```python
from build123d import *

# Parameters (mm, degrees)
BOSS_EXTRUDE1_DEPTH   = 7.9375
FILLET1_R             = 7.9375
SKETCH6_W             = 3.175
SKETCH6_H             = 7.9375
BOSS_EXTRUDE2_DEPTH   = 12.7
FILLET2_R             = 4.1275
FILLET3_R             = 4.1275
F_6_CLEARANCE_HOLE1_D = 4.3053


# Some blends are built 0.0001 mm under size
with BuildPart() as part:
    # Sketch1 → Boss-Extrude1 (new body)
    with BuildSketch(Plane(origin=(0, 0, 0), x_dir=(1, 0, 0), z_dir=(0, 1, 0))):
        Polygon((0, 0), (0, 22.225), (7.9375, 22.225), (7.9375, 50.45837), (11.1125, 50.45837), (11.1125, 19.05), (3.175, 19.05), (3.175, 0), align=None)
    extrude(amount=BOSS_EXTRUDE1_DEPTH)

    # Fillet1
    fillet1_edges = [part.edges().sort_by_distance(p)[0] for p in [
        (7.9375, 3.96875, -22.225),
        (3.175, 3.96875, -19.05),
    ]]
    fillet(fillet1_edges, radius=FILLET1_R - 0.0001)  # a hair under: the kernel refuses the full size

    # Sketch6 → Boss-Extrude2 (add)
    with BuildSketch(Plane(origin=(0, 7.9375, 0), x_dir=(1, 0, 0), z_dir=(0, 1, 0))):
        with Locations((9.525, 46.48962)):
            Rectangle(SKETCH6_W, SKETCH6_H)
    extrude(amount=BOSS_EXTRUDE2_DEPTH)

    # Fillet2
    # the kernel refuses this fillet: 4.1275 mm, written as the material it takes off along each edge
    with BuildSketch(Plane(origin=(21.43125, 20.6375, -50.45837), x_dir=(0, -1, 0), z_dir=(-1, 0, 0))) as fillet2_piece_1:
        with BuildLine():
            CenterArc((FILLET2_R, FILLET2_R), FILLET2_R, 180, 90)
            Line((0, FILLET2_R), (0, 0))
            Line((0, 0), (FILLET2_R, 0))
        make_face()
    extrude(amount=23.8125, mode=Mode.SUBTRACT)
    with BuildSketch(Plane(origin=(-2.38125, 20.6375, -42.52087), x_dir=(0, 0, -1), z_dir=(1, 0, 0))) as fillet2_piece_2:
        with BuildLine():
            CenterArc((FILLET2_R, -FILLET2_R), FILLET2_R, 90, 90)
            Line((0, -FILLET2_R), (0, 0))
            Line((0, 0), (FILLET2_R, 0))
        make_face()
    extrude(amount=23.8125, mode=Mode.SUBTRACT)

    # Fillet3
    fillet3_edges = [part.edges().sort_by_distance(p)[0] for p in [
        (9.525, 7.9375, -42.52087),
    ]]
    fillet(fillet3_edges, radius=FILLET3_R)

    # #6 Clearance Hole1 (through all)
    with Locations(Plane(origin=(0, 0, 0), x_dir=(0, 0, -1), z_dir=(-1, 0, 0))):
        with Locations((5.55625, -3.96875), (46.33087, -16.51)):
            Hole(F_6_CLEARANCE_HOLE1_D / 2)


solid = part.part
```
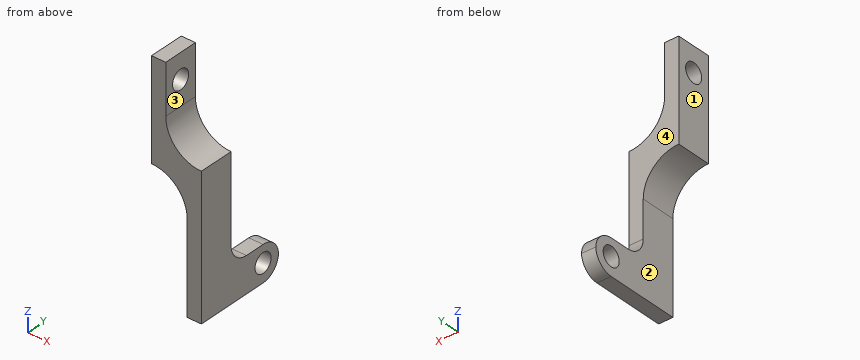
Part model, mm, in its own coordinate system. Face numbers are marked on the shaded views. A direction names the side the tool comes from. Coordinates: 2 decimals unless noted, no trailing zeros. Write each loop counter-clockwise with the first axis right and the second up, starting at its lowest first coordinate (ties: lowest second). Pieces come first, ordered by that corner, then holes.
Item 1: Which spindle directions (+Z, -Z, +X, -X, +Y, -Y) get a long thin tool onto all of the face, cutting with end or side? Do the marked faces 1, 2, 3 and 4. Say none if no direction does.
Item 2: Slice it at D-D (z = -34). Write the cut outline in (x, y), and give its area (3 significant figures).
Item 3: Probe line 1 (Z direction, x = 10.15, y = 16.51); line 2 (X direction, y = 7.5, z = -11) (3 decimals); line 3 (X direction, y = 5, z = -41.5). List the from-to ranges inside material, lowest first.
Item 4: Slice it at B-B (x = 9.5). Write the cut outline in (y, z) (1 decimal).
Item 5: Pin check, flat tips, straight feed: pin 1 (2.5 mm diameter, centred on x = 9, y = 14.5, fed in from +Z); pin 2 (2.5 mm diameter, centred on y = 16.51, z = -46.33, fed in from -X); pin 3 (5.5 mm diameter, centred on y = 3.97, z = -5.56, fed in from +X) (3 decimals); pin 4 (6 mm diameter, centred on x = 6.5, y = 12.5, fed in from +Z). Stop position of each tip, or through.
Results found:
1. face 1: +Z, -Z, -X, +Y, -Y
1. face 2: -Z, -X, +Y, -Y
1. face 3: +Z, +X, +Y, -Y
1. face 4: +Z, +X, -X, +Y
2. outline: (7.94, 0) - (11.11, 0) - (11.11, 7.94) - (7.94, 7.94) - close
2. area: 25.2 mm2
3. line 1: z = -50.46 to -48.48, -44.18 to -42.52
3. line 2: x = 0 to 3.175
3. line 3: x = 7.94 to 11.11
4. outline: (0, -50.5) - (16.5, -50.5) arc R4.1 ccw to (20.6, -46.5) arc R4.1 ccw to (16.5, -42.5) - (12.1, -42.5) arc R4.1 cw to (7.9, -38.4) - (7.9, -18.9) - (0, -18.9) - close; hole circle Ø4.3 at (16.5, -46.3)
5. pin 1: stops at z = -42.52
5. pin 2: passes through
5. pin 3: stops at x = 3.175
5. pin 4: stops at z = -41.89
